The listing builds one solid part. Answer for the finished solid, in the listing's coordinates (mm). A direction names the side the tool comes from. Give positions to 0.01 mm unless a question says otherwise; leave off trailing zeros. Loops run counter-clockwise (first coordinate to the right, second up) from the corner with the lowest first, then second, coordinate; pieces in that order, holes last. Notation, with made-up numbers: (79.25, -14) - (103.25, -14) arc R19 cw to (103.25, 18) - close; hole circle Ø11 at (-37.5, 87.5). An arc over 180 degrees is marked (long way). Answer in a Markdown table with one row per item. Add a question column.
```python
from build123d import *

# Parameters (mm, degrees)
SKETCH1_W           = 44.5
SKETCH1_H           = 40
BOSS_EXTRUDE1_DEPTH = 48.5
SKETCH2_W           = 39.5
SKETCH2_H           = 40
CUT_EXTRUDE1_DEPTH  = 46
FILLET1_R           = 1
SKETCH3_R           = 3
BOSS_EXTRUDE2_DEPTH = 2.5
SKETCH5_R           = 1.25
SKETCH5_R_2         = 5
CUT_EXTRUDE5_DEPTH  = 6
SKETCH7_R           = 4
CUT_EXTRUDE7_DEPTH  = 44.5
SKETCH8_R           = 1.25
CUT_EXTRUDE8_DEPTH  = 44.5
SKETCH9_W           = 44.5
SKETCH9_H           = 15
CUT_EXTRUDE9_DEPTH  = 10
SKETCH10_R          = 6
SKETCH10_R_2        = 5
EXTRUDE_THIN1_DEPTH = 20


with BuildPart() as part:
    # Sketch1 → Boss-Extrude1 (new body)
    with BuildSketch(Plane.XY):
        with Locations((22.25, 20)):
            Rectangle(SKETCH1_W, SKETCH1_H)
    extrude(amount=BOSS_EXTRUDE1_DEPTH)

    # Sketch2 → Cut-Extrude1 (cut)
    with BuildSketch(Plane.XY.offset(48.5)):
        with Locations((22.25, 20)):
            Rectangle(SKETCH2_W, SKETCH2_H)
    extrude(amount=-CUT_EXTRUDE1_DEPTH, mode=Mode.SUBTRACT)

    # Fillet1
    fillet1_edges = [part.edges().sort_by_distance(p)[0] for p in [
        (44.5, 20, 0),
        (0, 20, 0),
    ]]
    fillet(fillet1_edges, radius=FILLET1_R)

    # Sketch3 → Boss-Extrude2 (add)
    with BuildSketch(Plane.XY.offset(2.5)):
        with Locations((15.25, 19.5)):
            Circle(SKETCH3_R)
        with Locations((31.25, 19.5)):
            Circle(SKETCH3_R)
        with Locations((31.25, 35.5)):
            Circle(SKETCH3_R)
        with Locations((15.25, 35.5)):
            Circle(SKETCH3_R)
    extrude(amount=BOSS_EXTRUDE2_DEPTH)

    # Sketch5 → Cut-Extrude5 (cut)
    with BuildSketch(Plane.XY.offset(5)):
        with Locations((23.25, 35.5)):
            Circle(SKETCH5_R)
        with Locations((31.25, 35.5)):
            Circle(SKETCH5_R)
        with Locations((15.25, 35.5)):
            Circle(SKETCH5_R)
        with Locations((23.25, 27.5)):
            Circle(SKETCH5_R_2)
        with Locations((31.25, 27.5)):
            Circle(SKETCH5_R)
        with Locations((23.25, 19.5)):
            Circle(SKETCH5_R)
        with Locations((31.25, 19.5)):
            Circle(SKETCH5_R)
        with Locations((15.25, 27.5)):
            Circle(SKETCH5_R)
        with Locations((15.25, 19.5)):
            Circle(SKETCH5_R)
    extrude(amount=-CUT_EXTRUDE5_DEPTH, mode=Mode.SUBTRACT)

    # Sketch7 → Cut-Extrude7 (cut)
    with BuildSketch(Plane(origin=(44.5, 0, 0), x_dir=(0, 0, -1), z_dir=(1, 0, 0))):
        with Locations((-37.5, 12.5)):
            Circle(SKETCH7_R)
        with BuildLine():
            Line((-48.5, 40), (-48.5, 12.500000045))
            ThreePointArc((-48.5, 12.500000045), (-45.278174577, 20.278174609), (-37.5, 23.5))
            Line((-37.5, 23.5), (-1, 40))
            Line((-1, 40), (-48.5, 40))
        make_face()
        with BuildLine():
            ThreePointArc((-30.342192143, 4.147408386), (-33.684145427, 2.183059859), (-37.5, 1.5))
            ThreePointArc((-37.5, 1.5), (-45.278174609, 4.721825423), (-48.5, 12.500000045))
            Line((-48.5, 12.500000045), (-48.5, 0))
            Line((-48.5, 0), (-1, 0))
            Line((-1, 0), (-1, 15))
            Line((-1, 15), (-30.342192143, 4.147408386))
        make_face()
    extrude(amount=-CUT_EXTRUDE7_DEPTH, mode=Mode.SUBTRACT)

    # Sketch8 → Cut-Extrude8 (cut)
    with BuildSketch(Plane(origin=(44.5, 0, 0), x_dir=(0, 0, -1), z_dir=(1, 0, 0))):
        with Locations((-45.5, 12.5)):
            Circle(SKETCH8_R)
        with Locations((-37.5, 20.5)):
            Circle(SKETCH8_R)
        with Locations((-37.5, 4.5)):
            Circle(SKETCH8_R)
        with Locations((-29.5, 12.5)):
            Circle(SKETCH8_R)
    extrude(amount=-CUT_EXTRUDE8_DEPTH, mode=Mode.SUBTRACT)

    # Sketch9 → Cut-Extrude9 (cut)
    with BuildSketch(Plane.XY.offset(1)):
        with Locations((22.25, 7.5)):
            Rectangle(SKETCH9_W, SKETCH9_H)
    extrude(amount=-CUT_EXTRUDE9_DEPTH, mode=Mode.SUBTRACT)

    # Sketch10 → Extrude-Thin1 (add)
    with BuildSketch(Plane.XY.offset(2.5)):
        with Locations((23.25, 27.5)):
            Circle(SKETCH10_R)
        with Locations((23.25, 27.5)):
            Circle(SKETCH10_R_2, mode=Mode.SUBTRACT)
    extrude(amount=EXTRUDE_THIN1_DEPTH)


solid = part.part
```
(1) A cutting plane is placed at A-A on z = 14. Determine the outline of the cut face in (x, y), plus the area to 3 significant figures.
(2) A cutting plane is placed at C-C on y = 25.5. Determine the outline of the cut face in (x, z).
(3) The mould has two halves that part along X. Classify faces 1 (the face through (12.869, 17.675, 3.732)), 2 (the face through (0, 20, 19)), 3 (the face through (43.27, 19.74, 38.49)): pulls with the +X half, pulls with the -X half, needs draft (parallel to the pull), parting line crosses it, or undercut.
(4) Find the intervals of material crossed by line 1 along Y through (x, z) = (31.25, 3.25); line 2 along Y through (x, z) = (15.25, 0.7); line 3 along X through (y, z) = (7, 33.5), in increasing order. Write a range as [from, to].
(5) A tool of negligible diameter and unlimited length cuts with its end or side. For faces 4 (the face through (31.827, 18.391, 2.535)), 5 (the face through (31, 34, 5)), 6 (the face through (43.27, 3.74, 38.49)), 7 (the face through (2.5, 20, 21)), 8 (the face through (14.6, 32.57, 3.73)), from which of +Z, -Z, +X, -X, +Y, -Y can it reach the whole face along a straight path? Write none if from no direction.
(6) A cutting plane is placed at D-D on z = 27.5. Determine the outline of the cut face in (x, y), plus the area to 3 significant figures.
(7) Given pin 1 Ø6 at (x, y) = (23.25, 27.5) entering from -Z; pin 2 Ø9.5 at (x, y) = (20.5, 29) entering from +Z; pin 3 Ø1.1 at (x, z) = (16.5, 0.5) entering from -Y, each flat-ended and moving along its own axis, determine where each tip first touches the part or whether it passes through.
(8) A cutting plane is placed at B-B on x = 31.25. Determine the outline of the cut face in (y, z).
Evaluation:
| question | item | result |
|---|---|---|
| 1 | outline | (0, 10.19) - (2.5, 10.19) - (2.5, 34.12) - (0, 34.12) - close; circle Ø12 at (23.25, 27.5); (42, 10.19) - (44.5, 10.19) - (44.5, 34.12) - (42, 34.12) - close; hole circle Ø10 at (23.25, 27.5) |
| 1 | area | 154 mm² |
| 2 | outline | (0, 1) arc R1 ccw to (1, 0) - (18.67, 0) - (18.67, 22.5) - (17.59, 22.5) - (17.59, 2.5) - (2.5, 2.5) - (2.5, 33.08) - (0, 33.08) - close; (27.83, 0) - (43.5, 0) arc R1 ccw to (44.5, 1) - (44.5, 33.08) - (42, 33.08) - (42, 2.5) - (28.91, 2.5) - (28.91, 22.5) - (27.83, 22.5) - close |
| 3 | face 1 | undercut |
| 3 | face 2 | pulls with the -X half |
| 3 | face 3 | needs draft |
| 4 | line 1 | y = [16.5, 18.25], [20.75, 22.5], [32.5, 34.25], [36.75, 38.5] |
| 4 | line 2 | y = [15, 18.25], [20.75, 26.25], [28.75, 34.25], [36.75, 40] |
| 4 | line 3 | x = [0, 2.5], [42, 44.5] |
| 5 | face 4 | +Z, -Z |
| 5 | face 5 | +Z, +Y |
| 5 | face 6 | +X, -X |
| 5 | face 7 | +Z, +Y, -Y |
| 5 | face 8 | +Z |
| 6 | outline | (0, 5.2) - (2.5, 5.2) - (2.5, 28.02) - (0, 28.02) - close; (42, 5.2) - (44.5, 5.2) - (44.5, 28.02) - (42, 28.02) - close |
| 6 | area | 114 mm² |
| 7 | pin 1 | passes through |
| 7 | pin 2 | stops at z = 22.5 |
| 7 | pin 3 | stops at y = 14.98 |
| 8 | outline | (14.45, 2.5) - (15, 1) - (15, 0) - (18.25, 0) - (18.25, 5) - (16.5, 5) - (16.5, 2.5) - close; (20.75, 0) - (26.25, 0) - (26.25, 2.5) - (22.5, 2.5) - (22.5, 5) - (20.75, 5) - close; (28.75, 0) - (34.25, 0) - (34.25, 5) - (32.5, 5) - (32.5, 2.5) - (28.75, 2.5) - close; (36.75, 0) - (40, 0) - (40, 1) - (39.32, 2.5) - (38.5, 2.5) - (38.5, 4.32) - (38.19, 5) - (36.75, 5) - close |
